Job drawing, mm, ordinate dimensions from the low corner. One solid piece. A direction names the side the tool comes from. Coordinates: 2 decimals unless noted, no trailing zeros. Loops run counter-clockwise (first coordinate to the right, second up) from the corner with the lowest first, then second, coordinate; pieces in that order, holes last. Notation, with made-up numbers: (-10.75, 46.5) -> (20.25, 46.5) arc R20 ccw to (20.25, 68.5) -> close; hole circle Ø9 at (-6, 61.5). An arc over 180 degrees is marked (long way). Use one line per item in the form item = value. Start each with the question number.
(1) Drill centre lines: L1, parallel to Z at x = 20.75, y = 20.5; L2, parallel to X at y = 14, z = 27.5; L3, parallel to Y at x = 4, z = 36 (1 decimal). Where is each one in solid material? Low to high. Write a range as [from, to].
(2) Pin check, flat tips, straight feed: P1, Ø3, axis at x = 13.5, z = 28, coming from the +Y side; P2, Ø6, axis at x = 8, z = 12.5, coming from the +Y side; P3, Ø6, axis at x = 20.5, z = 16.5, coming from the +Y side (1 decimal). Stop position of each tip, or through.
(3) Band-saw the part on B-B on z = 32. Give the cut face in (x, y), then the cut area to 3 significant figures.
(4) 3-axis set-ups, long thin cutter, end or side, ignore diameter. For the marked faces 1 and 2: which of +Z, -Z, +X, -X, +Y, -Y reach the whole face in a straight line?
(5) Band-saw the part on A-A on z = 39. Give the cut face in (x, y) (1 decimal).
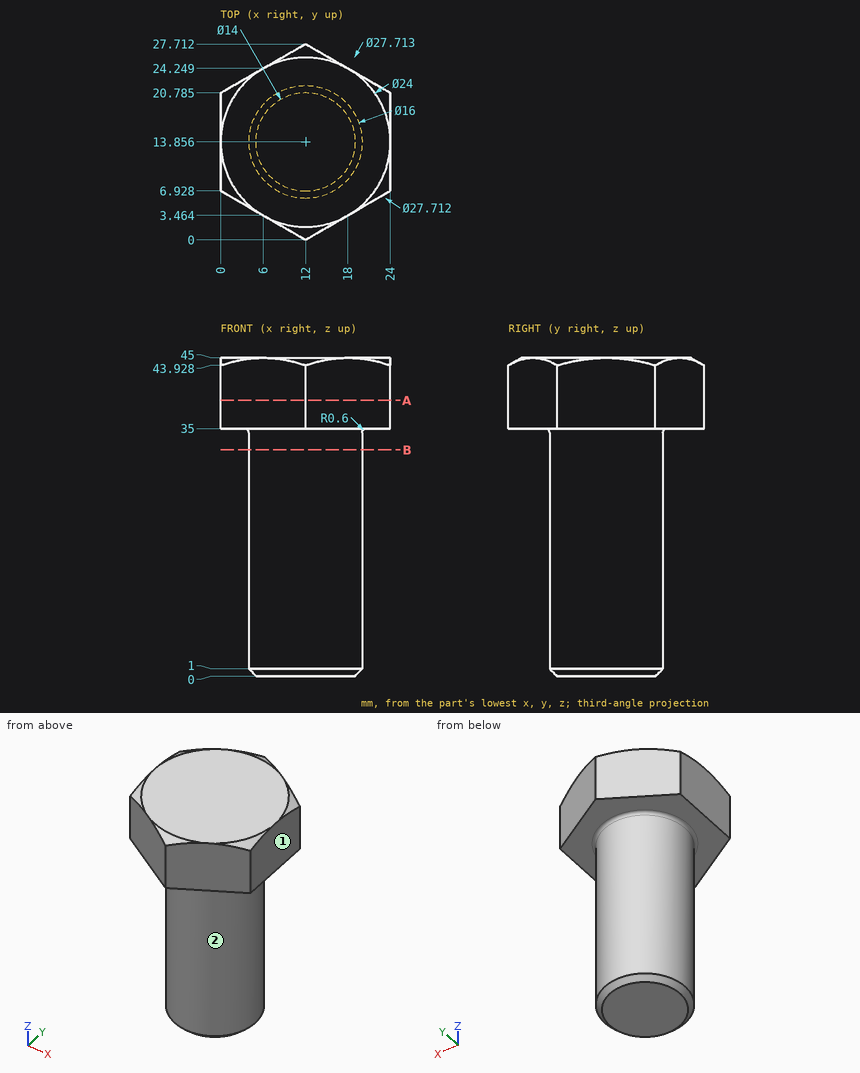
A:
q1.L1 = [35, 45]
q1.L2 = [4, 20]
q1.L3 = [4.6, 23.1]
q2.P1 = 21.86
q2.P2 = 21.79
q2.P3 = 19.7
q3.outline = circle Ø16 at (12, 13.86)
q3.area = 201 mm²
q4.face_1 = +Z, -Z, +X, +Y, -Y
q4.face_2 = -Z
q5.outline = (0, 6.9) -> (12, 0) -> (24, 6.9) -> (24, 20.8) -> (12, 27.7) -> (0, 20.8) -> close
